Can you work these out from the model? Positions are in its coordinate system, mm. A direction names the side the tool comes from. Round coordinates to 2 decimals unless told otherwise and drop trailing zeros. Order: outer loops, then holes, each group sorted by start corner. A loop starts at its lowest first (then second) coordinate and runs counter-clockwise, first axis right, second up.
Q1. If we section it at D-D (y = 6): Please give me the cut outline in (x, z), plus the area to 3 significant figures.
Q2. If I drill on line 1 (Y direction, x = 10.5, z = -50.1); line 2 (Z direction, x = 0, y = 1.25); line 3 (Z direction, x = 15, y = 22.5), over which ranges is the centre line in solid material (lowest first)?
Q3. For faces 1 (the face through (-6.2, 18, -51)), 2 (the face through (0, 1, 52.5)), 3 (the face through (-11.5, 1.5, -9.4)), 4 (the face through (0, 3, 1)), which set-ups out of +Z, -Z, +X, -X, +Y, -Y let a thin tool reach every point of the face, with its end or its side?
Q4. Will these pins go through, and if not, where does the flat tip stop? P1, Ø3, axis at x = -10.5, y = 27.4, coming from the +Z side; P2, Ø4, axis at x = -1.5, z = 10, coming from the +Y side.
Q5. If we section it at C-C (z = 13): Please give me the cut outline in (x, y).
Q6. If we section it at B-B (x = 1.5): Please give me the cut outline in (y, z), plus the area to 3 significant figures.
Q7. We'd pull the mould along X, two halves only. Please class faces 5 (the face through (0, 0, -1)), 6 (the face through (11.562, 14.46, -50.979)), 7 (the face through (-21.5, 2.7, -12.1)): pulls with the +X half, pulls with the -X half, needs draft (parallel to the pull), parting line crosses it, or undercut.
Q8. If we section it at A-A (y = 14.9): Please give me the cut outline in (x, z), plus the area to 3 significant figures.
Autodesk Fusion 360 part; units mm, degrees
sketch "Sketch1" plane through (0, 0, 0) normal (0, 1, 0) x (1, 0, 0)
  line L0 (21.5, 52.5) -> (-21.5, 52.5)
  line L1 (-21.5, 52.5) -> (-21.5, -52.5)
  line L2 (-21.5, -52.5) -> (21.5, -52.5)
  line L3 (21.5, -52.5) -> (21.5, 52.5)
  line L4 (21.5, 52.5) -> (-21.5, -52.5) construction
  line L5 (-21.5, 52.5) -> (21.5, -52.5) construction
  dimension "d1" = 43
  dimension "d2" = 105
extrude "Extrude1" add sketch "Sketch1" along normal blind 3
sketch "Sketch2" plane through (0, 3, 0) normal (0, 1, 0) x (-1, 0, 0)
  line L0 (-21.5, 52.5) -> (-21.5, -52.5)
  line L1 (-21.5, -52.5) -> (21.5, -52.5)
  line L2 (21.5, -52.5) -> (21.5, 52.5)
  line L3 (21.5, 52.5) -> (-21.5, 52.5)
  line L4 (15, -14.5) -> (-15, -14.5) construction
  line L5 (-15, -14.5) -> (-15, 50.5) construction
  line L6 (-15, 50.5) -> (15, 50.5) construction
  line L7 (15, 50.5) -> (15, -14.5) construction
  line L8 (-13.1, 47) -> (-13.1, 45)
  arc A0 (-13.1, 45) -> (-9.9, 45) centre (-11.5, 45) ccw
  line L9 (-9.9, 45) -> (-9.9, 47)
  arc A1 (-9.9, 47) -> (-13.1, 47) centre (-11.5, 47) ccw
  line L10 (-11.5, 47) -> (-11.5, 45) construction
  line L11 (0, 20) -> (0, 2.5)
  arc A2 (13.1, 47) -> (9.9, 47) centre (11.5, 47) ccw
  line L12 (13.1, 47) -> (13.1, 45)
  line L13 (9.9, 45) -> (9.9, 47)
  arc A3 (9.9, 45) -> (13.1, 45) centre (11.5, 45) ccw
  line L14 (-15, 18) -> (15, 18) construction
  arc A4 (-9.9, -11) -> (-13.1, -11) centre (-11.5, -11) ccw
  line L15 (-13.1, -11) -> (-13.1, -13)
  line L16 (-9.9, -13) -> (-9.9, -11)
  arc A5 (-13.1, -13) -> (-9.9, -13) centre (-11.5, -13) ccw
  line L17 (0, 1.75) -> (0, 22.5)
  line L18 (9.9, -13) -> (9.9, -11)
  arc A6 (13.1, -11) -> (9.9, -11) centre (11.5, -11) ccw
  line L19 (13.1, -11) -> (13.1, -13)
  arc A7 (9.9, -13) -> (13.1, -13) centre (11.5, -13) ccw
  dimension "d10" = 30
  dimension "d11" = 65
  dimension "d12" = 2
  dimension "d13" = 6.5
  dimension "d15" = 2
  dimension "d16" = 3.2
  dimension "d17" = 3.5
  dimension "d18" = 3.5
  dimension "d19" = 2
  dimension "d20" = 3.2
  dimension "d21" = 56
extrude "Extrude2" cut sketch "Sketch2" against normal blind 4 contours L8 A0 L9 A1 | A2 L12 L13 A3 | A4 L15 L16 A5 | L18 A6 L19 A7
sketch "Sketch3" plane through (0, 3, 0) normal (0, 1, 0) x (-1, 0, 0)
  line L0 (-9.9, -11) -> (-9.9, -13)
  arc A0 (-13.1, -13) -> (-9.9, -13) centre (-11.5, -13) ccw
  line L1 (-13.1, -13) -> (-13.1, -11)
  arc A1 (-9.9, -11) -> (-13.1, -11) centre (-11.5, -11) ccw
  line L2 (-13.1, 45) -> (-13.1, 47)
  arc A2 (-9.9, 47) -> (-13.1, 47) centre (-11.5, 47) ccw
  line L3 (-9.9, 47) -> (-9.9, 45)
  arc A3 (-13.1, 45) -> (-9.9, 45) centre (-11.5, 45) ccw
  line L4 (9.9, 45) -> (9.9, 47)
  arc A4 (13.1, 47) -> (9.9, 47) centre (11.5, 47) ccw
  line L5 (13.1, 47) -> (13.1, 45)
  arc A5 (9.9, 45) -> (13.1, 45) centre (11.5, 45) ccw
  line L6 (-21.5, 52.5) -> (-21.5, -52.5)
  line L7 (-21.5, -52.5) -> (21.5, -52.5)
  line L8 (21.5, -52.5) -> (21.5, 52.5)
  line L9 (21.5, 52.5) -> (-21.5, 52.5)
  line L10 (-21.5, -52.5) -> (21.5, -52.5)
  line L11 (21.5, -52.5) -> (21.5, -49.5)
  line L12 (21.5, -49.5) -> (-21.5, -49.5)
  line L13 (-21.5, -49.5) -> (-21.5, -52.5)
  line L14 (9.9, -13) -> (9.9, -11)
  arc A6 (13.1, -11) -> (9.9, -11) centre (11.5, -11) ccw
  line L15 (13.1, -11) -> (13.1, -13)
  arc A7 (9.9, -13) -> (13.1, -13) centre (11.5, -13) ccw
  dimension "d24" = 3
extrude "Extrude3" add sketch "Sketch3" along normal blind 28 contours L6 L7 L8 L10 L11 L12 L13
sketch "Sketch4" plane through (0, 0, -49.5) normal (0, 0, 1) x (1, 0, 0)
  line L0 (-21.5, 3) -> (21.5, 3)
  line L1 (21.5, 3) -> (21.5, 31)
  line L2 (21.5, 31) -> (-21.5, 31)
  line L3 (-21.5, 31) -> (-21.5, 3)
  line L4 (6.2, 27.4) -> (-6.2, 27.4)
  line L5 (-6.2, 27.4) -> (-6.2, 9)
  line L6 (-6.2, 9) -> (6.2, 9)
  line L7 (6.2, 9) -> (6.2, 27.4)
  line L8 (0, 2.5) -> (0, 20)
  line L9 (-10.5, 27.4) -> (10.5, 27.4) construction
  circle A0 centre (-10.5, 27.4) radius 1.15
  circle A1 centre (10.5, 27.4) radius 1.15
  line L10 (-10.5, 14.9) -> (10.5, 14.9) construction
  circle A2 centre (-10.5, 14.9) radius 1.15
  circle A3 centre (10.5, 14.9) radius 1.15
  line L11 (-6.2, 18.2) -> (6.2, 18.2)
  circle A4 centre (10.5, 9) radius 1.15
  circle A5 centre (-10.5, 21.5) radius 1.15
  circle A6 centre (-10.5, 9) radius 1.15
  circle A7 centre (10.5, 21.5) radius 1.15
  line L12 (6.2, 27.4) -> (6.2, 9)
  line L13 (-6.2, 27.4) -> (6.2, 27.4)
  line L14 (-6.2, 9) -> (-6.2, 27.4)
  line L15 (6.2, 9) -> (-6.2, 9)
  dimension "d27" = 12.4
  dimension "d28" = 6.2
  dimension "d29" = 18.4
  dimension "d30" = 6
  dimension "d33" = 2.3
  dimension "d34" = 2.3
  dimension "d35" = 12.5
  dimension "d38" = 2.3
  dimension "d39" = 2.3
  dimension "d40" = 21
  dimension "d41" = 21
  dimension "d42" = 10.5
extrude "Extrude4" cut sketch "Sketch4" against normal up to surface (3 mm away) contours L5 L6 L8 L11 L14 L15 | L6 L7 L8 L11 L12 L15 | L4 L5 L7 L11 L12 L13 L14 | A0 | A1 | A2 | A3 | A4 | A5 | A6 | A7
sketch "Sketch5" plane through (0, 3, 0) normal (0, 1, 0) x (-1, 0, 0)
  line L0 (-21.5, 52.5) -> (-21.5, -49.5)
  line L1 (-21.5, -49.5) -> (21.5, -49.5)
  line L2 (21.5, -49.5) -> (21.5, 52.5)
  line L3 (-9.9, -11) -> (-9.9, -13)
  arc A0 (-13.1, -13) -> (-9.9, -13) centre (-11.5, -13) ccw
  line L4 (-13.1, -13) -> (-13.1, -11)
  arc A1 (-9.9, -11) -> (-13.1, -11) centre (-11.5, -11) ccw
  line L5 (-13.1, 45) -> (-13.1, 47)
  arc A2 (-9.9, 47) -> (-13.1, 47) centre (-11.5, 47) ccw
  line L6 (-9.9, 47) -> (-9.9, 45)
  arc A3 (-13.1, 45) -> (-9.9, 45) centre (-11.5, 45) ccw
  line L7 (9.9, 45) -> (9.9, 47)
  arc A4 (13.1, 47) -> (9.9, 47) centre (11.5, 47) ccw
  line L8 (13.1, 47) -> (13.1, 45)
  arc A5 (9.9, 45) -> (13.1, 45) centre (11.5, 45) ccw
  circle A6 centre (0, -34.5) radius 3.5
  line L9 (9.9, -13) -> (9.9, -11)
  arc A7 (13.1, -11) -> (9.9, -11) centre (11.5, -11) ccw
  line L10 (13.1, -11) -> (13.1, -13)
  arc A8 (9.9, -13) -> (13.1, -13) centre (11.5, -13) ccw
  line L11 (21.5, 52.5) -> (-21.5, 52.5)
  dimension "d49" = 7
  dimension "d55" = 15
extrude "Extrude6" cut sketch "Sketch5" against normal up to surface (3 mm away) contours A6
fillet "Fillet3" radius 0.6 4 edges at (21.5, 1.5, 52.5) (-21.5, 1.5, 52.5) (-21.5, 31, -51) (21.5, 31, -51)
Solution:
1. outline: (-21.5, -52.5) - (21.5, -52.5) - (21.5, -49.5) - (-21.5, -49.5) - close
1. area: 129 mm2
2. line 1: y = 0 to 7.85, 10.15 to 13.75, 16.05 to 20.35, 22.65 to 26.25, 28.55 to 31
2. line 2: z = -52.5 to -38, -31 to 52.5
2. line 3: z = -52.5 to -49.5
3. face 1: +Z, -Z
3. face 2: +Z, +X, -X, +Y, -Y
3. face 3: +Y, -Y
3. face 4: +Z, +X, -X, +Y
4. P1: stops at z = -49.5
4. P2: stops at y = 3
5. outline: (-21.5, 0) - (21.5, 0) - (21.5, 3) - (-21.5, 3) - close
6. outline: (0, -52.5) - (9, -52.5) - (9, -49.5) - (3, -49.5) - (3, -37.66) - (0, -37.66) - close; (0, -31.34) - (3, -31.34) - (3, 52.5) - (0, 52.5) - close; (27.4, -52.5) - (31, -52.5) - (31, -49.5) - (27.4, -49.5) - close
6. area: 325 mm2
7. face 5: needs draft
7. face 6: undercut
7. face 7: pulls with the -X half
8. outline: (-21.5, -52.5) - (-11.65, -52.5) - (-11.65, -49.5) - (-21.5, -49.5) - close; (-9.35, -52.5) - (-6.2, -52.5) - (-6.2, -49.5) - (-9.35, -49.5) - close; (6.2, -52.5) - (9.35, -52.5) - (9.35, -49.5) - (6.2, -49.5) - close; (11.65, -52.5) - (21.5, -52.5) - (21.5, -49.5) - (11.65, -49.5) - close
8. area: 78.0 mm2
